The listing builds one solid part. Answer for the finished solid, in the listing's coordinates (mm). A direction names the side the tool comes from. Round coordinates to 2 decimals unless told otherwise and drop trailing zeros. Write each question's results on one line, items separated by ' | '. Start each with the question number.
from build123d import *

# Parameters (mm, degrees)
F1_DEPTH      = 70
F2_R          = 7.5
F3_DEPTH      = 70
F4_W          = 38.3359060888
F4_H          = 25
F4_W_2        = 39.5979748373
F4_W_3        = 30.4998038337
F4_H_2        = 20
F5_DEPTH      = 25
F5_DEPTH_BACK = 25
F6_R          = 15
F7_W          = 61.4808317696
F7_H          = 11.3357962312
F7_R          = 4.225
F8_DEPTH      = 70
F9_W          = 100
F9_H          = 20
F10_DEPTH     = 24
F11_R         = 2.125
F12_DEPTH     = 70
F14_R         = 2.125
F15_DEPTH     = 10


with BuildPart() as f1:
    # F0 (on Front) → F1 (new body)
    with BuildSketch(Plane.XZ):
        with BuildLine():
            add(Edge.make_bspline(
                [(0, 7.5), (50.3453426063, 33.0532751977), (124.5695498707, 70.4313359242), (325.5609958993, 110.9176804755), (447.3313093185, 59.5129579306), (600, 13.1103944731)],
                knots=[0, 0, 0, 0, 0.281013924, 0.5871772284, 1, 1, 1, 1], degree=3))
            ThreePointArc((0, 7.5), (-11.0976940951, -8.2685881847), (5.0424365564, -18.8186294225))
            add(Edge.make_bspline(
                [(5.0424365564, -18.8186294225), (104.1736466206, 0.0529713977), (299.4595954862, 54.136097737), (497.3786234374, 6.3046680419), (596.6067802216, -12.6636686144)],
                knots=[0, 0, 0, 0, 0.4997002441, 1, 1, 1, 1], degree=3))
            ThreePointArc((596.6067802216, -12.6636686144), (612.9982332309, -1.7112498691), (600, 13.1103944731))
        make_face()
    extrude(amount=F1_DEPTH)

    # F2 (on Front) → F3 (cut)
    with BuildSketch(Plane.XZ):
        with Locations((3.1568240374, -5.3793457337)):
            Circle(F2_R)
        with Locations((599.981546402, 0)):
            Circle(F2_R)
    extrude(amount=F3_DEPTH, mode=Mode.SUBTRACT)

    # F4 (on Top) → F5 (cut, two sides)
    with BuildSketch(Plane.XY) as f5_sk:
        with Locations((594.4681697192, -12.5)):
            Rectangle(F4_W, F4_H)
        with Locations((593.837135345, -57.5)):
            Rectangle(F4_W_2, F4_H)
        with Locations((3.3916295506, -35)):
            Rectangle(F4_W_3, F4_H_2)
    extrude(amount=-F5_DEPTH, mode=Mode.SUBTRACT)
    extrude(f5_sk.sketch, amount=F5_DEPTH_BACK, mode=Mode.SUBTRACT)

    # F6
    f6_edges = [f1.edges().sort_by_distance(p)[0] for p in [
        (574.038148, -57.5, -8.276448),
        (575.300217, -12.5, -8.524983),
    ]]
    fillet(f6_edges, radius=F6_R)

    # F7 (on Front) → F8 (join)
    with BuildSketch(Plane.XZ):
        with Locations((271.9227431553, 24.7699965359)):
            Rectangle(F7_W, F7_H)
        with BuildLine():
            Line((302.6631590401, 19.1020984203), (241.1823272705, 19.1020984203))
            ThreePointArc((241.1823272705, 19.1020984203), (271.9227431553, -11.6383174646), (302.6631590401, 19.1020984203))
        make_face()
        with Locations((271.9227431553, 9.1020984203)):
            Circle(F7_R, mode=Mode.SUBTRACT)
    extrude(amount=F8_DEPTH)

    # F9 (on Top) → F10 (cut)
    with BuildSketch(Plane.XY):
        with Locations((278, -35)):
            Rectangle(F9_W, F9_H)
    extrude(amount=F10_DEPTH, mode=Mode.SUBTRACT)

    # F11 (on Front) → F12 (join)
    with BuildSketch(Plane.XZ):
        with BuildLine():
            Line((472.1937120855, 53.3293670855), (510.3209194065, 41.2333121589))
            ThreePointArc((510.3209194065, 41.2333121589), (497.2994567763, 66.3263890307), (472.1937120855, 53.3293670855))
        make_face()
        with Locations((494.275441611, 56.7945826814)):
            Circle(F11_R, mode=Mode.SUBTRACT)
        Polygon((509.0549868975, 37.4887385523), (510.3209194065, 41.2333121589), (472.1937120855, 53.3293670855), (471.0067243804, 49.6005392228), align=None)
    extrude(amount=F12_DEPTH)

    # F14 (on offset) → F15 (cut)
    with BuildSketch(Plane(origin=(0, -30, 0), x_dir=(-1, 0, 0), z_dir=(0, 1, 0))):
        with BuildLine():
            ThreePointArc((-472.1937120855, 53.3293670855), (-497.2994567763, 66.3263890307), (-510.3209194065, 41.2333121589))
            Line((-510.3209194065, 41.2333121589), (-472.1937120855, 53.3293670855))
        make_face()
        with Locations((-494.275441611, 56.7945826814)):
            Circle(F14_R, mode=Mode.SUBTRACT)
    extrude(amount=-F15_DEPTH, mode=Mode.SUBTRACT)


solid = f1.part
Item 1: Straight lines are drawn through the part: L1, parallel to Y at x = 250, z = 3; L2, parallel to Z at x = 440, y = -50; L3, parallel to Z at x = 501.5, y = -9. For each, find the intervals that lie inside material, in ascending order. Write a range as [from, to].
Item 2: Determine the mould class of faces 1 (the flat face through (492, -30, 54)), 2 (the flat face through (591, -25, 4)), 3 (the cylindrical face through (-2.795, -12.325, -9.943)) for opening direction Y: +Y half, -Y half, draft (parallel to the pull), parting line (faces both ways), or undercut.
Item 3: For faces 4 (the flat face through (18.642, -35, 0)), 5 (the flat face through (271, -45, 14)), 6 (the flat face through (302.663, -35, 25)), 7 (the flat face through (492, -40, 54)), 8 (the flat face through (574.038, -58, 15)), determine the directions among +Z, -Z, +X, -X, +Y, -Y from which every point of the face is accessible in a straight line to the end or side of a thin tool.
Item 4: Each of these flat-tipped pins is pushed along its axis until it touches: pin 1 Ø6 at (y, z) = (-34, 13.5) entering from +X; pin 2 Ø4.5 at (y, z) = (-51.5, 21.5) entering from -X; pin 3 Ø5.5 at (y, z) = (-58.5, 16) entering from +X. Where does it stop, or does it pass through?
Item 5: The part is cut by section A-A, the plane y = -18.5. Give the number of separate pieces and of enclosed holes in the cut face, plus the area to 3 significant figures.
Report:
1) L1: y = [-70, -45], [-25, 0] | L2: z = [16.99, 63.38] | L3: z = [6.06, 64.44]
2) face 1: undercut | face 2: +Y half | face 3: draft
3) face 4: +Z, -Z, -X | face 5: none | face 6: -Z, +Y, -Y | face 7: +Z, +X | face 8: +Z, -Z, +X, -Y
4) pin 1: stops at x = 607.85 | pin 2: stops at x = 23.24 | pin 3: stops at x = 574.04
5) separate pieces: 1 | enclosed holes: 3 | area: 32,000 mm2
